```python
from build123d import *

# Parameters (mm, degrees)
EXTRUDE_1_DEPTH     = 5
SKETCH_2_R          = 1.6
CUT_EXTRUDE_1_DEPTH = 76.007176866
SKETCH_3_R          = 1.6
CUT_EXTRUDE_2_DEPTH = 6
CUT_EXTRUDE_3_DEPTH = 2
FILLET_1_R          = 1
EXTRUDE_2_DEPTH     = 1
FILLET_2_R          = 1.5
FILLET_3_R          = 10


with BuildPart() as part:
    # 草图1 → 凸台-拉伸1 (new, symmetric)
    with BuildSketch(Plane.XY):
        with BuildLine():
            Line((-41.92820323, 12), (-17.92820323, 53.569219382))
            Line((-17.92820323, 53.569219382), (-23.124355653, 56.569219382))
            Line((-23.124355653, 56.569219382), (-47.124355653, 15))
            ThreePointArc((-47.124355653, 15), (-47.94437584, 2.666789511), (-38.674353195, -5.509223834))
            Line((-38.674353195, -5.509223834), (-11.2624538, -12.96494456))
            ThreePointArc((-11.2624538, -12.96494456), (-10.39273309, -12.794497892), (-10, -12))
            Line((-10, -12), (-10, -6))
            Line((-10, -6), (10, -6))
            Line((10, -6), (10, 0))
            Line((10, 0), (-35, 0))
            ThreePointArc((-35, 0), (-41.92820323, 4), (-41.92820323, 12))
        make_face()
    extrude(amount=EXTRUDE_1_DEPTH, both=True)

    # 草图2 → 切除-拉伸1 (cut, through all)
    with BuildSketch(Plane(origin=(0, 0, 0), x_dir=(1, 0, 0), z_dir=(0, 1, 0))):
        with Locations(Location((0, 0, 0), (0, 0, 180))):
            Circle(SKETCH_2_R)
    extrude(amount=-CUT_EXTRUDE_1_DEPTH, mode=Mode.SUBTRACT)

    # 草图3 → 切除-拉伸2 (cut)
    with BuildSketch(Plane(origin=(-41.838457268, 24.155444566, 0), x_dir=(0, 0, 1), z_dir=(-0.8660254037844367, 0.5000000000000036, 0))):
        with Locations(Location((0, 32.42820323, 0), (0, 0, 270))):
            Circle(SKETCH_3_R)
        with Locations(Location((0, -5.57179677, 0), (0, 0, 270))):
            Circle(SKETCH_3_R)
    extrude(amount=-CUT_EXTRUDE_2_DEPTH, mode=Mode.SUBTRACT)

    # 草图4 → 切除-拉伸3 (cut)
    with BuildSketch(Plane(origin=(-36.642304845, 21.155444566, 0), x_dir=(0, 0, -1), z_dir=(0.8660254037844365, -0.5000000000000039, 0))):
        Polygon((1.58771324, 35.17820323), (-1.58771324, 35.17820323), (-3.175426481, 32.42820323), (-1.58771324, 29.67820323), (1.58771324, 29.67820323), (3.175426481, 32.42820323), align=None)
        Polygon((1.58771324, -2.82179677), (-1.58771324, -2.82179677), (-3.175426481, -5.57179677), (-1.58771324, -8.32179677), (1.58771324, -8.32179677), (3.175426481, -5.57179677), align=None)
    extrude(amount=-CUT_EXTRUDE_3_DEPTH, mode=Mode.SUBTRACT)

    # 圆角1
    fillet_1_edges = [part.edges().sort_by_distance(p)[0] for p in [
        (10, -3, -5),
        (-20.526279442, 55.069219382, -5),
        (-20.526279442, 55.069219382, 5),
        (10, -3, 5),
    ]]
    fillet(fillet_1_edges, radius=FILLET_1_R)

    # 草图6 → 凸台-拉伸2 (add, symmetric)
    with BuildSketch(Plane.XY):
        with BuildLine():
            Line((-41.92820323, 12), (-40.856406461, 13.856406461))
            Line((-40.856406461, 13.856406461), (-27, 0))
            Line((-27, 0), (-35, 0))
            ThreePointArc((-35, 0), (-41.92820323, 4), (-41.92820323, 12))
        make_face()
    extrude(amount=EXTRUDE_2_DEPTH, both=True)

    # 圆角2
    fillet_2_edges = [part.edges().sort_by_distance(p)[0] for p in [
        (-10, -6, 0),
    ]]
    fillet(fillet_2_edges, radius=FILLET_2_R)

    # 圆角3
    fillet_3_edges = [part.edges().sort_by_distance(p)[0] for p in [
        (-27, 0, 0),
    ]]
    fillet(fillet_3_edges, radius=FILLET_3_R)


solid = part.part
```
Can you work these out from the model? Positions are in its coordinate system, mm. A direction names the side the tool comes from. Give positions to 0.01 mm unless a question says otherwise; leave off trailing zeros. Order: outer loops, then holes, each group sorted by start corner. A loop starts at its lowest first (then second) coordinate and runs counter-clockwise, first axis right, second up. Notation, with made-up numbers: M -40,34.5 L 19,34.5 A11 cw 19,39.5 Z; hole C -12,-30.5 d10. An arc over 180 degrees is marked long. Write item = value, one per line. Start each with the question number.
Q1. Suppose I cut it at C-C (y = 37). Write out the boundary of the cut face in (x, z).
Q2. We'd pull the mould along Z, two halves only. Please class faces 1 (the flat face through (-37, 5, -1)), 2 (the flat face through (-37, 5, 1)), 3 (the flat face through (-20.58, 50.94, 2.37)), 4 (the flat face through (-20.49, 55.05, 0.06)): pulls with the +Z half, pulls with the -Z half, needs draft (parallel to the pull), parting line crosses it, or undercut.
Q3. Will these pins go through, and if not, where does the flat tip stop? pin 1 Ø4 at (x, z) = (-15, 3.5) entering from -Y; pin 2 Ø3 at (y, z) = (-0.5, -3) entering from -X; pin 3 Ø5 at (x, z) = (-1, -1.5) entering from -Y; pin 4 Ø11 at (x, y) = (-37.5, 6.5) entering from -Z.
Q4. Suppose I cut it at D-D (x = -7.5). Write out the boundary of the cut face in (y, z), plus the area to 3 significant figures.
Q5. Suppose I cut it at A-A (x = 0). Write out the boundary of the cut face in (y, z), plus the area to 3 significant figures.
Q6. For faces 5 (the flat face through (-22.66, 47.35, 0.02)), 6 (the flat face through (-19.907, 52.114, -0.022)), 7 (the flat face through (3, -6, 0)), 8 (the cylindrical face through (-41.87, 3.9, 3.03)), which set-ups out of +Z, -Z, +X, -X, +Y, -Y let a thin tool reach every point of the face, with its end or its side?
Q7. I need wall thicknesses on probe 1 along Z at (x, y) = (0, -2); probe 2 along Y at (x, z) = (-24, -3); probe 3 along X at (y, z) = (24, 1). Which ranges of each line are inside material? Lowest first, please. Write a range as [from, to].
Q8. Suppose I cut it at B-B (z = 0). Count the separate pieces of the cut face and the enclosed holes in it, plus the area to 3 significant figures.
Check result:
q1.outline = M -34.42,-5 L -27.49,-5 L -27.49,5 L -34.42,5 Z
q2.face_1 = pulls with the -Z half
q2.face_2 = pulls with the +Z half
q2.face_3 = undercut
q2.face_4 = needs draft
q3.pin_1 = -12.49
q3.pin_2 = -47.12
q3.pin_3 = -6
q3.pin_4 = -5
q4.outline = M -6,-5 L 0,-5 L 0,5 L -6,5 Z
q4.area = 60.0 mm2
q5.outline = M -6,-5 L 0,-5 L 0,-1.6 L -6,-1.6 Z; M -6,1.6 L 0,1.6 L 0,5 L -6,5 Z
q5.area = 40.8 mm2
q6.face_5 = +X
q6.face_6 = none
q6.face_7 = +Z, -Z, +X, -Y
q6.face_8 = +Z, +X
q7.probe_1 = [-5, -1.6], [1.6, 5]
q7.probe_2 = [-9.5, 0], [43.05, 55.05]
q7.probe_3 = [-41.93, -35]
q8.separate_pieces = 4
q8.enclosed_holes = 0
q8.area = 838 mm2
